Can you work these out from the model? Positions are in its coordinate system, mm. A direction names the side the tool comes from. Round coordinates to 2 decimals unless told otherwise and drop trailing zeros. Loops run counter-clockwise (first coordinate to the right, second up) from the corner with the lowest first, then second, coordinate; pieces in that order, holes last.
Autodesk Inventor part; units mm, degrees
ref_plane "stopper_to_body_XY" through (0, 0, 0) normal (0, 0, 1) x (1, 0, 0)
ref_plane "stopper_to_body_YZ" through (0, 0, 0) normal (1, 0, 0) x (0, 1, 0)
ref_plane "stopper_to_body_ZX" through (0, 0, 0) normal (0, 1, 0) x (0, 0, 1)
sketch "Sketch_1" plane through (0, 0, 0) normal (0, 0, 1) x (1, 0, 0)
  line L0 (-28.4294, 25.5589) -> (-24.6062, 23.3516)
  arc A0 (-24.6062, 23.3516) -> (-16.9438, 4.0925) centre (-8.5838, 18.5724) ccw
  line L1 (-16.9438, 4.0925) -> (-14.9819, 2.9597)
  arc A1 (-14.5696, 2.4169) -> (-14.9819, 2.9597) centre (-15.4219, 2.1976) ccw
  arc A2 (-14.5696, 2.4169) -> (-13.7753, 0) centre (4.18, 7.24) ccw
  arc A3 (-13.7753, 0) -> (0, -11.6634) centre (4.18, 7.24) ccw
  arc A4 (0, -11.6634) -> (9.3779, -11.4092) centre (4.18, 7.24) ccw
  arc A5 (10.0541, -11.4948) -> (9.3779, -11.4092) centre (9.6141, -12.2569) ccw
  line L2 (10.0541, -11.4948) -> (12.0161, -12.6275)
  arc A6 (12.0161, -12.6275) -> (32.5262, -9.6338) centre (20.3761, 1.8524) ccw
  line L3 (32.5262, -9.6338) -> (36.3494, -11.8411)
  line L4 (36.3494, -11.8411) -> (37.2294, -10.3169)
  line L5 (37.2294, -10.3169) -> (15.1777, 2.4147)
  arc A7 (13.4621, 4.218) -> (15.1777, 2.4147) centre (17.3777, 6.2252) ccw
  arc A8 (13.4621, 4.218) -> (-3.0781, 13.7676) centre (-2.2, -3.8105) ccw
  arc A9 (-5.4977, 14.3516) -> (-3.0781, 13.7676) centre (-3.2977, 18.1621) ccw
  line L6 (-5.4977, 14.3516) -> (-27.5494, 27.0831)
  line L7 (-27.5494, 27.0831) -> (-28.4294, 25.5589)
  line L8 (19.8, -12.32) -> (24.2, -12.32)
  line L9 (24.2, -12.32) -> (24.2, -7.04)
  arc A10 (24.2, -7.04) -> (23.76, -6.6) centre (23.76, -7.04) ccw
  line L10 (23.76, -6.6) -> (20.24, -6.6)
  arc A11 (20.24, -6.6) -> (19.8, -7.04) centre (20.24, -7.04) ccw
  line L11 (19.8, -7.04) -> (19.8, -12.32)
  arc A12 (-14.2873, 14.8537) -> (-14.1263, 14.2526) centre (-13.9063, 14.6337) ccw
  line L12 (-14.1263, 14.2526) -> (-11.0778, 12.4926)
  arc A13 (-11.0778, 12.4926) -> (-10.4768, 12.6537) centre (-10.8578, 12.8737) ccw
  line L13 (-10.4768, 12.6537) -> (-9.3768, 14.5589)
  line L14 (-9.3768, 14.5589) -> (-13.1873, 16.7589)
  line L15 (-13.1873, 16.7589) -> (-14.2873, 14.8537)
extrude "Extrusion1" add sketch "Sketch_1" along normal blind 25
sketch "Sketch_2" plane through (0, 0, 2.3) normal (0, 0, 1) x (1, 0, 0)
  line L0 (-29.3094, 24.0347) -> (-25.4862, 21.8274)
  arc A0 (-25.4862, 21.8274) -> (-17.8238, 2.5683) centre (-9.4638, 17.0482) ccw
  line L1 (-17.8238, 2.5683) -> (-15.8619, 1.4355)
  arc A1 (-15.4496, 0.8927) -> (-15.8619, 1.4355) centre (-16.3019, 0.6734) ccw
  arc A2 (-15.4496, 0.8927) -> (-14.6553, -1.5242) centre (3.3, 5.7158) ccw
  arc A3 (-14.6553, -1.5242) -> (-0.88, -13.1876) centre (3.3, 5.7158) ccw
  arc A4 (-0.88, -13.1876) -> (8.4979, -12.9334) centre (3.3, 5.7158) ccw
  line L2 (8.4979, -12.9334) -> (8.4979, 7.921)
  arc A5 (8.4979, 7.921) -> (-3.9581, 12.2434) centre (-3.08, -5.3347) ccw
  arc A6 (-6.3777, 12.8274) -> (-3.9581, 12.2434) centre (-4.1777, 16.6379) ccw
  line L3 (-6.3777, 12.8274) -> (-28.4294, 25.5589)
  line L4 (-28.4294, 25.5589) -> (-29.3094, 24.0347)
extrude "Extrusion2" cut sketch "Sketch_2" along normal blind 50
sketch "Sketch_8" plane through (0, 0, 4.6) normal (0, 0, 1) x (1, 0, 0)
  line L0 (8.4979, 7.921) -> (8.4979, -12.9334)
  arc A0 (9.1741, -13.019) -> (8.4979, -12.9334) centre (8.7341, -13.7811) ccw
  line L1 (9.1741, -13.019) -> (11.1361, -14.1517)
  arc A1 (11.1361, -14.1517) -> (31.6462, -11.158) centre (19.4961, 0.3282) ccw
  line L2 (31.6462, -11.158) -> (35.4694, -13.3653)
  line L3 (35.4694, -13.3653) -> (36.3494, -11.8411)
  line L4 (36.3494, -11.8411) -> (14.2977, 0.8905)
  arc A2 (12.5821, 2.6938) -> (14.2977, 0.8905) centre (16.4977, 4.701) ccw
  arc A3 (12.5821, 2.6938) -> (8.4979, 7.921) centre (-3.08, -5.3347) ccw
extrude "Extrusion3" cut sketch "Sketch_8" along normal blind 50
sketch "Sketch_9" plane through (0, 0, 0) normal (0, 0, 1) x (1, 0, 0)
  line L0 (9.3779, 11.6892) -> (9.3779, -11.4092)
  arc A0 (10.0541, -11.4948) -> (9.3779, -11.4092) centre (9.6141, -12.2569) ccw
  line L1 (10.0541, -11.4948) -> (12.0161, -12.6275)
  arc A1 (12.0161, -12.6275) -> (32.5262, -9.6338) centre (20.3761, 1.8524) ccw
  line L2 (32.5262, -9.6338) -> (36.3494, -11.8411)
  line L3 (36.3494, -11.8411) -> (38.1094, -8.7927)
  line L4 (38.1094, -8.7927) -> (16.0577, 3.9389)
  arc A2 (14.3421, 5.7423) -> (16.0577, 3.9389) centre (18.2577, 7.7494) ccw
  arc A3 (14.3421, 5.7423) -> (9.3779, 11.6892) centre (-1.32, -2.2863) ccw
  line L5 (19.8, -12.32) -> (24.2, -12.32)
  line L6 (24.2, -12.32) -> (24.2, -7.04)
  arc A4 (24.2, -7.04) -> (23.76, -6.6) centre (23.76, -7.04) ccw
  line L7 (23.76, -6.6) -> (20.24, -6.6)
  arc A5 (20.24, -6.6) -> (19.8, -7.04) centre (20.24, -7.04) ccw
  line L8 (19.8, -7.04) -> (19.8, -12.32)
extrude "Extrusion4" cut sketch "Sketch_9" along normal blind 2.3
sketch "Sketch_3" plane through (0, 0, 0) normal (0.5, 0.866, 0) x (0.866, -0.5, 0)
  line L0 (-80, -90) -> (80, -90)
  line L1 (80, -90) -> (80, 10)
  line L2 (80, 10) -> (-80, 10)
  line L3 (-80, 10) -> (-80, -90)
  line L4 (-37.4, -8) -> (-37.4, -15)
  arc A0 (-37.4, -15) -> (-32.4, -20) centre (-32.4, -15) ccw
  line L5 (-32.4, -20) -> (-31.6329, -20)
  arc A1 (-31.6329, -20) -> (-28.8967, -19.5175) centre (-31.6329, -12) ccw
  line L6 (-28.8967, -19.5175) -> (-4.3403, -10.5797)
  arc A2 (3.5382, -11.9689) -> (-4.3403, -10.5797) centre (-1.6041, -18.0973) ccw
  line L7 (3.5382, -11.9689) -> (16.8375, -23.1284)
  arc A3 (16.8375, -23.1284) -> (21.9798, -25) centre (21.9798, -17) ccw
  line L8 (21.9798, -25) -> (25.4, -25)
  arc A4 (25.4, -25) -> (37.4, -13) centre (25.4, -13) ccw
  line L9 (37.4, -13) -> (37.4, -12)
  arc A5 (37.4, -12) -> (25.4, 0) centre (25.4, -12) ccw
  line L10 (25.4, 0) -> (-29.4, 0)
  arc A6 (-29.4, 0) -> (-37.4, -8) centre (-29.4, -8) ccw
extrude "Extrusion5" cut sketch "Sketch_3" along normal mid plane 100
sketch "Sketch_7" plane through (0, 0, 0) normal (1, 0, 0) x (0, 1, 0)
  line L0 (0, 0) -> (0, 8)
  line L1 (0, 8) -> (4, 8)
  arc A0 (6, 6) -> (4, 8) centre (4, 6) ccw
  line L2 (6, 6) -> (6, 5)
  line L3 (6, 5) -> (0, 5)
  line L4 (0, 5) -> (0, 8)
sketch "Sketch_4" plane through (0, 0, 2.3) normal (0, 0, 1) x (1, 0, 0)
  arc A0 (-3.5, -7.5) -> (3.5, -7.5) centre (0, -7.5) ccw
  line L0 (3.5, -7.5) -> (3.5, 7.5)
  arc A1 (3.5, 7.5) -> (-3.5, 7.5) centre (0, 7.5) ccw
  line L1 (-3.5, 7.5) -> (-3.5, -7.5)
extrude "Extrusion6" add sketch "Sketch_4" along normal blind 2.7
revolve "Revolution1" add sketch "Sketch_7" angle 360 about axis through (0, 0, 0) along (0, 0, -1)
ref_plane "stopper_to_body_XY" through (0, 0, 0) normal (0, 0, 1) x (1, 0, 0)
ref_plane "stopper_to_body_YZ" through (0, 0, 0) normal (1, 0, 0) x (0, 1, 0)
ref_plane "stopper_to_body_ZX" through (0, 0, 0) normal (0, 1, 0) x (0, 0, 1)
properties part number "STOPPER-HSMCS50"
(1) If we mould it in two halves opening along X, with no side actions, what happens to faces 1 (the cylindrical face through (-8.23, -7.62, 1.13)), 2 (the flat face through (33.14, -9.99, 3.85)), 3 (the flat face through (25, -4, 25)), 4 (the flat face through (22, -12.32, 3))? For each: released by +X, released by -X, zero draft, split by the parting line, or undercut.
Worked answers:
face 1: released by -X
face 2: undercut
face 3: zero draft
face 4: undercut
(2) For faces 5 (the flat face through (-13.73, 15.82, 1.13)), 6 (the flat face through (-3.5, 0, 4)), 7 (the cylindrical face through (13.32, 1.66, 11.71)), 8 (the flat face through (0, 0, 8)), which set-ups out of +Z, -Z, +X, -X, +Y, -Y let a thin tool reach every point of the face, with its end or its side?
Worked answers:
face 5: +Z, -Z
face 6: -X, -Y
face 7: +Z, -Y
face 8: +Z, -X, -Y
(3) If we section it at A-A, the plane x = 11: List the corners of the cut face in (y, z) for me, then the cut area to 3 significant figures.
Worked answers:
outline: (-12.04, 2.3) - (7.83, 2.3) - (7.83, 13.71) - (5.23, 14.8) - (5.23, 4.6) - (-12.04, 4.6) - close
area: 70.9 mm2
(4) Will these pins go through, and if not, where does the flat tip stop? P1, Ø3, axis at x = -5.5, y = -0.5, coming from the -Z side; P2, Ø2, axis at y = 2, z = 3, coming from the +X side; P3, Ø5, axis at y = 15, z = 13, coming from the -X side; P4, Ø2.5, axis at x = -1, y = 0.5, coming from the +Z side.
Worked answers:
P1: stops at z = 0
P2: stops at x = 17.63
P3: stops at x = -14.47
P4: stops at z = 8
(5) If I drill on line 1 (Z direction, x = -3, y = 2.5); line 2 (Z direction, x = 13, y = -7.5); line 3 (X direction, y = -6.5, z = 22), over which ranges is the centre line in solid material (lowest first)?
Worked answers:
line 1: z = 0 to 8
line 2: z = 2.3 to 4.6
line 3: x = 27.1 to 30.62
